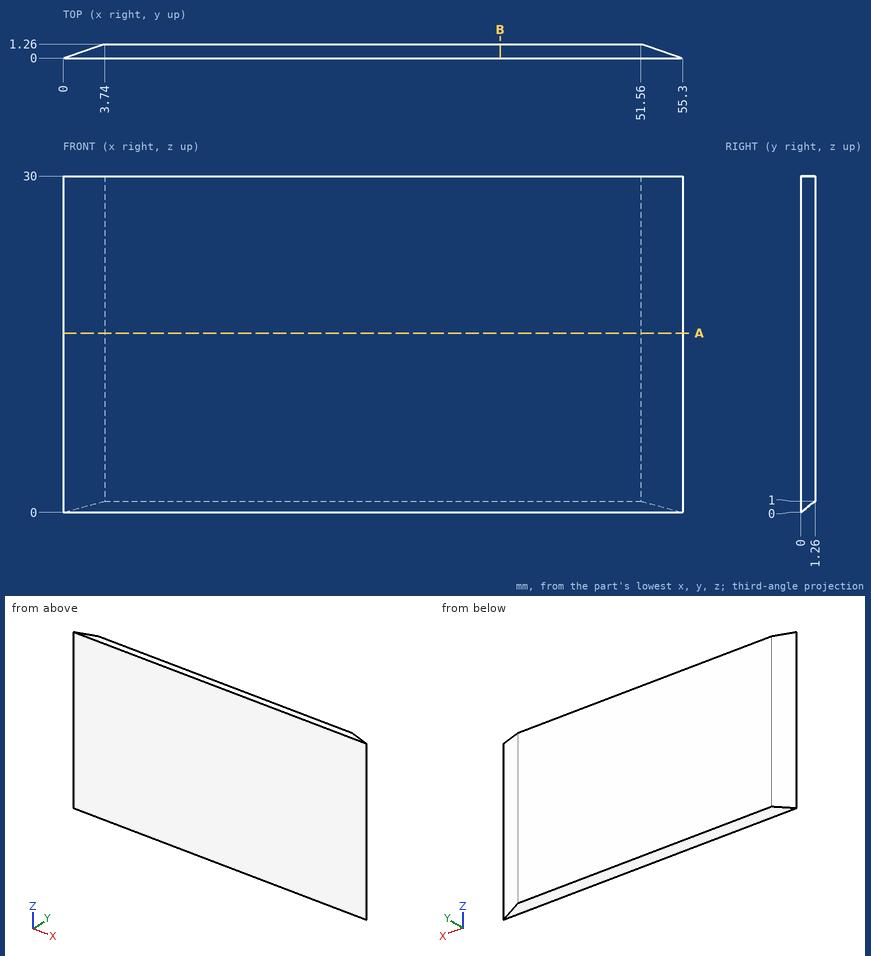
The figure shows three views and two pictorial views of one solid part (mm, origin at its lowest corner). Answer the questions. Round coordinates to 2 decimals unless told otherwise and drop trailing zeros. Loops run counter-clockwise (first coordinate to the right, second up) from the corner with the lowest first, then second, coordinate; pieces in that order, holes last. Notation, with made-up numbers: M -27.5,-22.75 L 11.5,-22.75 A26 cw 11.5,3.25 Z; hole C 36,71 d10. An arc over 180 degrees is marked long. Use CSV: the item, a comma, the result in double quotes.
Q1. Section B-B, the plane x = 39 is taken. Determine the outline of the cut face in (y, z).
Determined:
outline,"M 0,0 L 1.26,1 L 1.26,30 L 0,30 Z"
Q2. Consider L1, parallel to Z at x = 35, y = 0.85; L2, parallel to Z at x = 44.5, y = 0.2; L3, parallel to Y at x = 52, z = 6. Determine where each line is inside the solid, lowest interval first.
Determined:
L1,"0.67 to 30"
L2,"0.16 to 30"
L3,"0 to 1.11"
Q3. Section A-A, the plane z = 16 is taken. Determine the outline of the cut face in (x, y), then the cut area to 3 significant figures.
Determined:
outline,"M 0,0 L 55.3,0 L 51.56,1.26 L 3.74,1.26 Z"
area,"65.0 mm2"
